Job drawing, mm, ordinate dimensions from the low corner. One solid piece. Round coordinates to 2 decimals unless told otherwise and drop trailing zeros. Loops run counter-clockwise (first coordinate to the right, second up) from the corner with the lowest first, then second, coordinate; pieces in that order, holes last. Notation, with made-up numbers: M 65,-5.5 L 93,-5.5 A18 cw 93,29.5 Z; hole C 4.25,-28 d10. An arc over 180 degrees is marked long. Use one line per item in the form item = value.
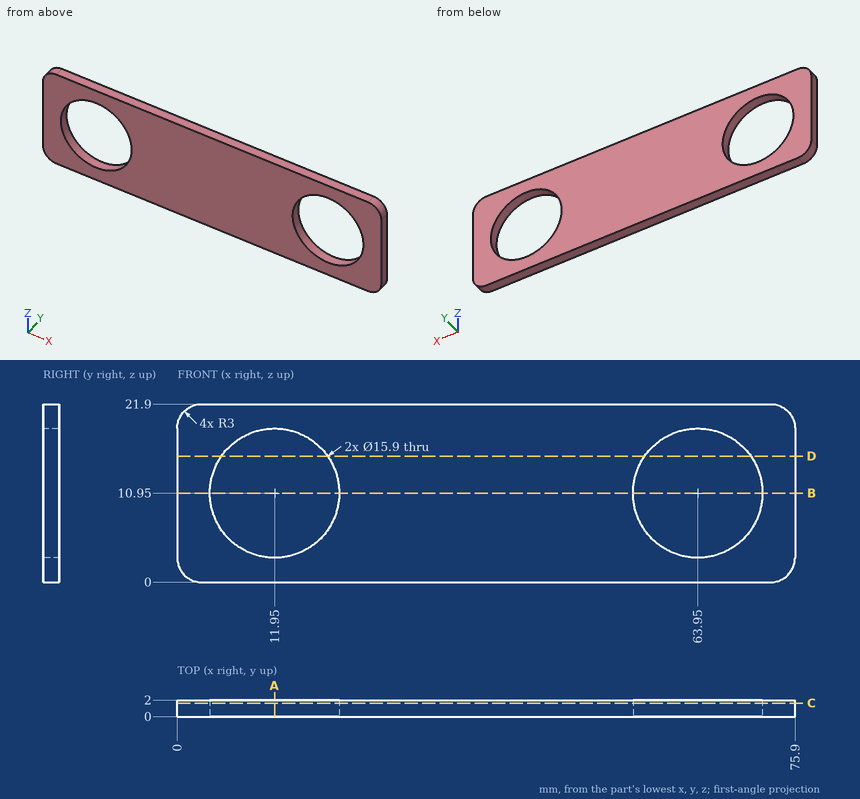
1. Cut at B-B on z = 10.95. Write the cut outline in (x, y).
Completed:
outline = M 0,0 L 4,0 L 4,2 L 0,2 Z; M 19.9,0 L 56,0 L 56,2 L 19.9,2 Z; M 71.9,0 L 75.9,0 L 75.9,2 L 71.9,2 Z
2. Probe line 1 along X through (y, z) = (1.25, 10.95); line 2 along Z through (x, y) = (7.5, 0.65); line 3 along Z through (x, y) = (57, 0.9). List the from-to ranges inside material, lowest first. Write a range as from..to.
Completed:
line_1 = 0..4, 19.9..56, 71.9..75.9
line_2 = 0..4.36, 17.54..21.9
line_3 = 0..7.09, 14.81..21.9
3. Cut at C-C on y = 1.65. Write the cut outline in (x, z), and give its area (3 significant figures).
Completed:
outline = M 0,3 A3 ccw 3,0 L 72.9,0 A3 ccw 75.9,3 L 75.9,18.9 A3 ccw 72.9,21.9 L 3,21.9 A3 ccw 0,18.9 Z; hole C 11.95,10.95 d15.9; hole C 63.95,10.95 d15.9
area = 1,260 mm2
4. Cut at D-D on z = 15.5. Write the cut outline in (x, y), and give its area (3 significant figures).
Completed:
outline = M 0,0 L 5.43,0 L 5.43,2 L 0,2 Z; M 18.47,0 L 57.43,0 L 57.43,2 L 18.47,2 Z; M 70.47,0 L 75.9,0 L 75.9,2 L 70.47,2 Z
area = 99.6 mm2
5. Cut at A-A on x = 11.95. Write the cut outline in (y, z), and give its area (3 significant figures).
Completed:
outline = M 0,0 L 2,0 L 2,3 L 0,3 Z; M 0,18.9 L 2,18.9 L 2,21.9 L 0,21.9 Z
area = 12.0 mm2
